from build123d import *

# Parameters (mm, degrees)
F0_W     = 34.925
F0_H     = 63.5
F1_DEPTH = 34.925
F2_W     = 6.35
F2_H     = 9.525
F3_DEPTH = 38.1
F4_R     = 3.175
F5_DEPTH = 34.926
F6_R     = 3.175
F7_DEPTH = 25.4
F8_R     = 6.35


with BuildPart() as f1:
    # F0 (on Top) → F1 (new body)
    with BuildSketch(Plane.XY):
        Rectangle(F0_W, F0_H)
    extrude(amount=F1_DEPTH)

    # F2 (on face) → F3 (cut)
    with BuildSketch(Plane(origin=(0, 31.75, 0), x_dir=(-1, 0, 0), z_dir=(0, 1, 0))):
        with Locations((-14.2875, 30.1625)):
            Rectangle(F2_W, F2_H)
        with Locations((-14.2875, 4.7625)):
            Rectangle(F2_W, F2_H)
        with Locations((14.2875, 30.1625)):
            Rectangle(F2_W, F2_H)
        with Locations((14.2875, 4.7625)):
            Rectangle(F2_W, F2_H)
        Polygon((11.1125, 34.925), (-11.1125, 34.925), (-11.1125, 25.4), (-11.1125, 9.525), (-11.1125, 0), (11.1125, 0), (11.1125, 9.525), (11.1125, 25.4), align=None)
    extrude(amount=-F3_DEPTH, mode=Mode.SUBTRACT)

    # F4 (on face) → F5 (cut, through all)
    with BuildSketch(Plane(origin=(-17.4625, 0, 0), x_dir=(0, -1, 0), z_dir=(-1, 0, 0))):
        with Locations((-22.225, 17.4625)):
            Circle(F4_R)
    extrude(amount=-F5_DEPTH, mode=Mode.SUBTRACT)

    # F6 (on face) → F7 (cut)
    with BuildSketch(Plane.XZ.offset(31.75)):
        with Locations((0, 17.4625)):
            Circle(F6_R)
    extrude(amount=-F7_DEPTH, mode=Mode.SUBTRACT)

    # F8
    f8_edges = [f1.edges().sort_by_distance(p)[0] for p in [
        (14.2875, 31.75, 25.4),
        (14.2875, -6.35, 25.4),
        (-14.2875, -6.35, 25.4),
        (-14.2875, 31.75, 25.4),
        (-14.2875, 31.75, 9.525),
        (14.2875, 31.75, 9.525),
        (14.2875, -6.35, 9.525),
        (-14.2875, -6.35, 9.525),
        (11.1125, -6.35, 17.4625),
        (-11.1125, -6.35, 17.4625),
    ]]
    fillet(f8_edges, radius=F8_R)


solid = f1.part
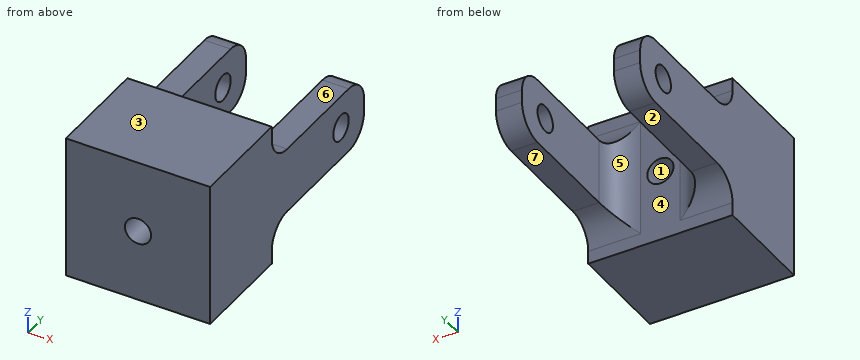
Read the model definition and answer for the solid it produces. Units are mm, in the model's axes. Face numbers are marked on the shaded views. A direction names the side the tool comes from. Give positions to 0.01 mm unless a question says otherwise; leave off trailing zeros. Write each loop counter-clockwise with the first axis right and the second up, starting at its lowest first coordinate (ties: lowest second). Pieces come first, ordered by that corner, then holes. Notation, with made-up numbers: (86, 4) -> (111, 4) arc R20 cw to (111, 22) -> close; hole circle Ø1 at (56.25, 51.25). An arc over 180 degrees is marked (long way). Answer as a JSON object with one key per item and string values. Group by question number.
1) Find section D-D (z = 15). Write down the section's boundary in (x, y), and give its area (3 significant figures).
2) The mould has two halves that part along Z. Classify the marked faces 1, 2 and 3: +Z half, -Z half, draft (parallel to the pull), parting line (faces both ways), or undercut.
3) A tool of negligible diameter and unlimited length cuts with its end or side. For the marked faces 4, 5, 6 and 7, from which of +Z, -Z, +X, -X, +Y, -Y can it reach the whole face along a straight path? Write none if from no direction.
4) Each of these flat-tipped pins is pushed along its axis until it touches: P1, Ø1.5, axis at x = 12, z = 4.5, coming from the +Y side; P2, Ø1.5, axis at x = -1.5, z = 25, coming from the +Y side; P3, Ø5, axis at x = 8.5, y = 20.5, coming from the -Z side; P4, Ø3, axis at x = -10, z = 12, coming from the +Y side (3 decimals). Where does it stop, or does it pass through?
5) Consider L1, parallel to X at y = 27, z = 14.5; L2, parallel to Z at x = 0, y = -20 (1 decimal); L3, parallel to Z at x = 11.5, y = 20.5 (3 decimals). Determine where each line is inside the solid, lowest interval first. Write a range as from..to.
6) Find section B-B (y = 1). Write down the section's boundary in (x, z) (1 decimal).
Values follow:
{
 "1": {"outline": "(-17.46, -31.75) -> (-2, -31.75) -> (-2, -6.35) -> (-4.76, -6.35) arc R6.35 cw to (-11.11, 0) -> (-11.11, 20.22) -> (-17.46, 20.22) -> close; (-17.46, 24.23) -> (-11.11, 24.23) -> (-11.11, 31.69) -> (-17.46, 31.69) -> close; (2, -31.75) -> (17.46, -31.75) -> (17.46, 20.22) -> (11.11, 20.22) -> (11.11, 0) arc R6.35 cw to (4.76, -6.35) -> (2, -6.35) -> close; (11.11, 24.23) -> (17.46, 24.23) -> (17.46, 31.69) -> (11.11, 31.69) -> close", "area": "1,230 mm2"},
 "2": {"face 1": "undercut", "face 2": "-Z half", "face 3": "+Z half"},
 "3": {"face 4": "+Y", "face 5": "+Z, -Z, +Y", "face 6": "+Z, +X, -X, +Y", "face 7": "-Z, +X, -X, +Y"},
 "4": {"P1": "stops at y = -6", "P2": "stops at y = -6.35", "P3": "passes through", "P4": "stops at y = 31.065"},
 "5": {"L1": "x = -17.46..-11.11, 11.11..17.46", "L2": "z = 0..14.3, 20.6..34.9", "L3": "z = 9.525..14.797, 20.128..25.4"},
 "6": {"outline": "(-17.5, 9.5) -> (-11.1, 9.5) -> (-11.1, 25.4) -> (-17.5, 25.4) -> close; (11.1, 9.5) -> (17.5, 9.5) -> (17.5, 25.4) -> (11.1, 25.4) -> close"}
}
